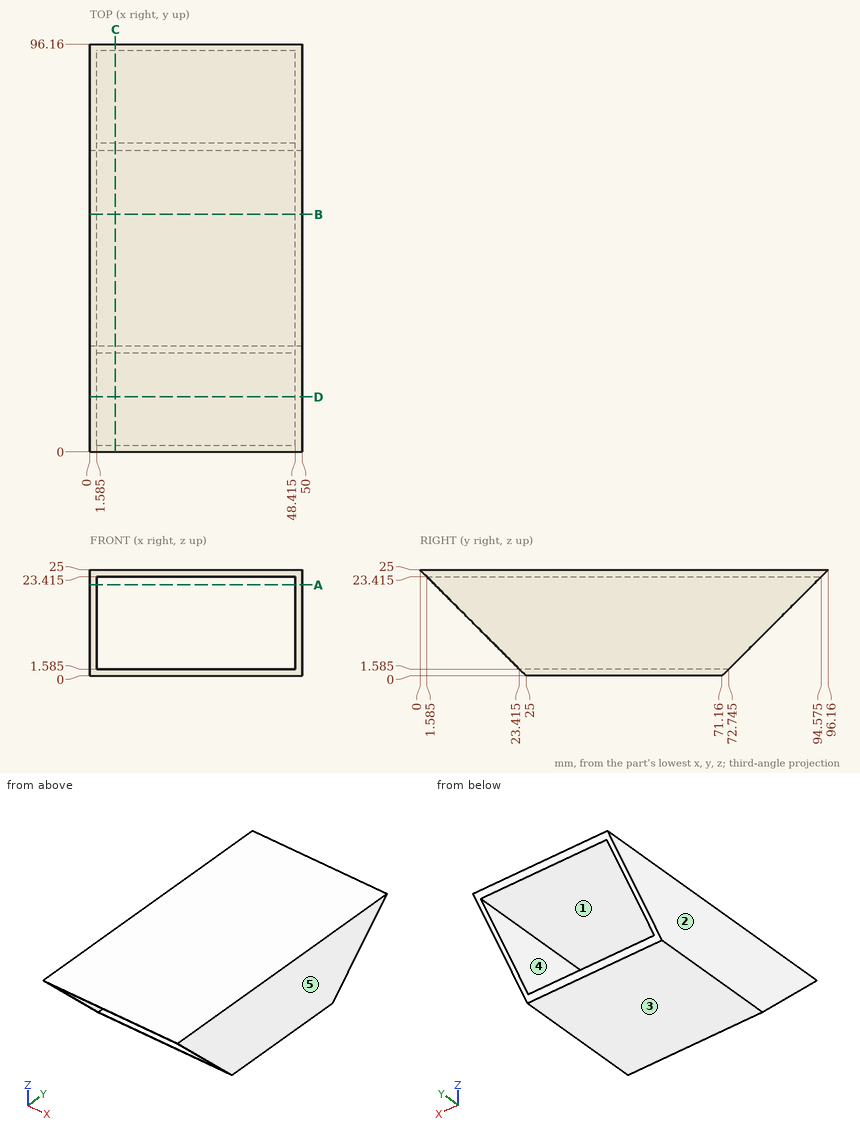
Job drawing, mm, ordinate dimensions from the low corner. One solid piece. A direction names the side the tool comes from. Give positions to 0.01 mm unless a question says otherwise; leave off trailing zeros. Order: outer loops, then holes, each group sorted by start corner. A loop starts at its lowest first (then second) coordinate and runs counter-clockwise, first axis right, second up. Notation, with made-up numbers: (55, 37.25) - (63, 37.25) arc R26 cw to (63, 68.25) - close; hole circle Ø8 at (85.5, 86). An arc over 180 degrees is marked (long way). Answer in a Markdown table with one row per item.
1. Saw through at C-C, the plane x = 6. Give the cut face in (y, z) (3 decimals).
Data:
| item | result |
|---|---|
| outline | (0, 25) - (1.585, 23.415) - (94.575, 23.415) - (96.16, 25) - close; (23.415, 1.585) - (25, 0) - (71.16, 0) - (72.745, 1.585) - close |
2. Probe probe 1 along X at (y, z) = (21, 9.5) (3 decimals); probe 2 along Z at (x, y) = (14, 60) (3 decimals); probe 3 along Z at (x, y) = (20, 82) (3 decimals). List the from-to ranges inside material, lowest first. Write a range as [from, to].
Data:
| item | result |
|---|---|
| probe 1 | x = [0, 1.585], [48.415, 50] |
| probe 2 | z = [0, 1.585], [23.415, 25] |
| probe 3 | z = [23.415, 25] |
3. Tool access for the marked faces 4 and 5: list every direction of +Z, -Z, +X, -X, +Y, -Y with a clear straight run to the whole face (end or side of a thin tool).
Data:
| item | result |
|---|---|
| face 4 | +Y, -Y |
| face 5 | +Z, -Z, +X, +Y, -Y |
4. Pull direction Z, two halves, no side cores. Call the marked faces 1, 2 and 3: pulls with the +Z half, pulls with the -Z half, needs draft (parallel to the pull), parting line crosses it, or undercut.
Data:
| item | result |
|---|---|
| face 1 | undercut |
| face 2 | needs draft |
| face 3 | pulls with the -Z half |
5. Saw through at B-B, the plane y = 56. Give the cut face in (x, z) (3 decimals), plus the area to 3 significant figures.
Data:
| item | result |
|---|---|
| outline | (0, 0) - (50, 0) - (50, 25) - (0, 25) - close; hole (1.585, 1.585) - (48.415, 1.585) - (48.415, 23.415) - (1.585, 23.415) - close |
| area | 228 mm² |
6. Flat gauge pin, fed straight in: pin 1 (11 mm diameter, centred on y = 33.5, z = 12, fed in from -X). Where does the tip first touch, or does it go through?
Data:
| item | result |
|---|---|
| pin 1 | stops at x = 0 |
7. Saw through at D-D, the plane y = 13. Give the cut face in (x, z) (3 decimals), plus the area to 3 significant figures.
Data:
| item | result |
|---|---|
| outline | (0, 12) - (1.585, 12) - (1.585, 23.415) - (48.415, 23.415) - (48.415, 12) - (50, 12) - (50, 25) - (0, 25) - close |
| area | 115 mm² |
8. Saw through at A-A, the plane z = 21.5. Give the cut face in (x, y) (3 decimals).
Data:
| item | result |
|---|---|
| outline | (0, 3.5) - (1.585, 3.5) - (1.585, 92.66) - (0, 92.66) - close; (48.415, 3.5) - (50, 3.5) - (50, 92.66) - (48.415, 92.66) - close |
